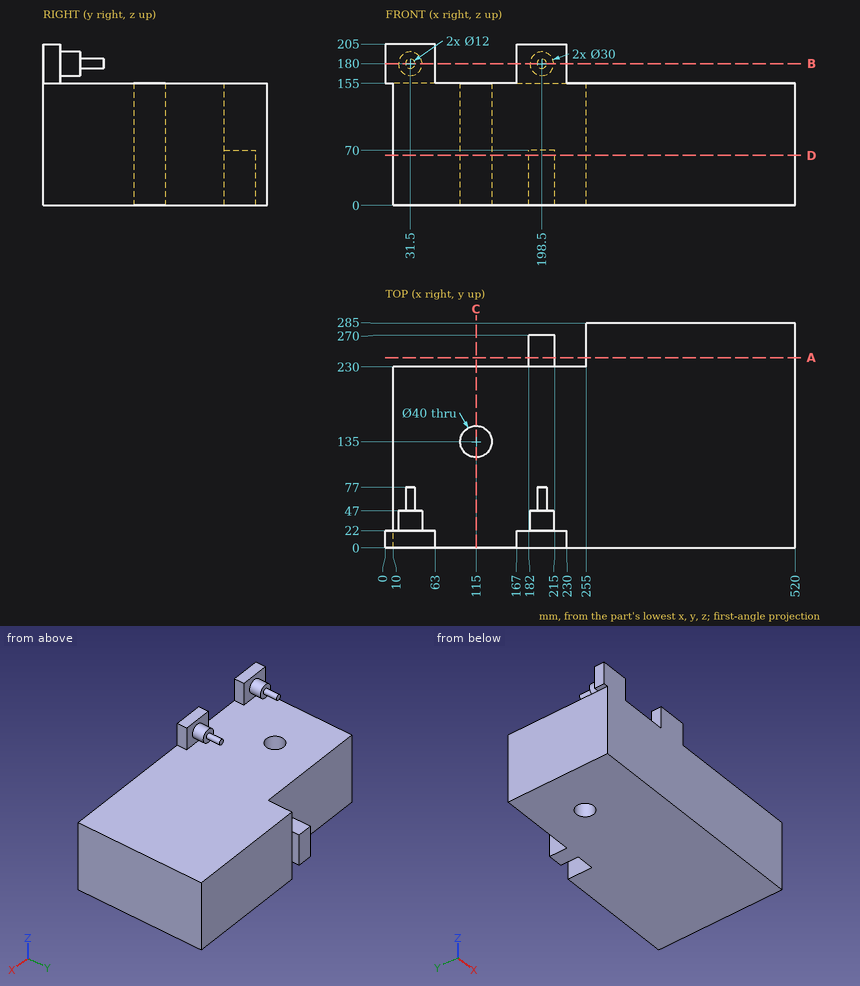
Here's the drawing with two shaded views (mm, measured from the low corner). I have some questions. Round coordinates to 2 decimals unless told otherwise and drop trailing zeros. Order: outer loops, then holes, each group sorted by start corner. A loop starts at its lowest first (then second) coordinate and runs counter-clockwise, first axis right, second up. Notation, with made-up numbers: (61, 85) -> (105, 85) arc R16 ccw to (105, 104) -> close; hole circle Ø8 at (73, 14). An arc over 180 degrees is marked (long way). Return JSON: item names as keys, results as strings.
Q1. If we section it at D-D on z = 63.5: List the corners of the cut face in (x, y) for me.
Filled sheet:
{"outline": "(10, 0) -> (520, 0) -> (520, 285) -> (255, 285) -> (255, 230) -> (215, 230) -> (215, 270) -> (182, 270) -> (182, 230) -> (10, 230) -> close; hole circle Ø40 at (115, 135)"}
Q2. I need wall thicknesses on line 1 along Y through (x, z) = (115, 75.5); line 2 along Z through (x, y) = (499.5, 121.5); line 3 along X through (y, z) = (201, 148.5). Which ranges of each line are inside material? Lowest first, please. Write a range as from..to.
Filled sheet:
{"line 1": "y = 0..115, 155..230", "line 2": "z = 0..155", "line 3": "x = 10..520"}
Q3. If we section it at A-A on y = 241.5: List the corners of the cut face in (x, z) for me, plus the area to 3 significant figures.
Filled sheet:
{"outline": "(182, 0) -> (215, 0) -> (215, 70) -> (182, 70) -> close; (255, 0) -> (520, 0) -> (520, 155) -> (255, 155) -> close", "area": "43,400 mm^2"}
Q4. For pin 1 Ø9.5 at (x, z) = (33, 178.5) entering from +Y; pin 2 Ø16.5 at (x, y) = (193.5, 255) entering from +Z; pin 3 Ø20 at (y, z) = (256.5, 23.5) entering from -X; pin 4 Ø3 at (x, z) = (237, 82) entering from -Y, each with a flat end and sliding along its axis, tell me the tip position at first contact or that it passes through.
Filled sheet:
{"pin 1": "stops at y = 77", "pin 2": "stops at z = 70", "pin 3": "stops at x = 182", "pin 4": "stops at y = 0"}
Q5. If we section it at C-C on x = 115: List the corners of the cut face in (y, z) for me, plus the area to 4 significant figures.
Filled sheet:
{"outline": "(0, 0) -> (115, 0) -> (115, 155) -> (0, 155) -> close; (155, 0) -> (230, 0) -> (230, 155) -> (155, 155) -> close", "area": "29,450 mm^2"}
Q6. If we section it at B-B on z = 180: List the corners of the cut face in (x, y) for me, plus the area to 3 significant figures.
Filled sheet:
{"outline": "(0, 0) -> (63, 0) -> (63, 22) -> (46.5, 22) -> (46.5, 47) -> (37.5, 47) -> (37.5, 77) -> (25.5, 77) -> (25.5, 47) -> (16.5, 47) -> (16.5, 22) -> (0, 22) -> close; (167, 0) -> (230, 0) -> (230, 22) -> (213.5, 22) -> (213.5, 47) -> (204.5, 47) -> (204.5, 77) -> (192.5, 77) -> (192.5, 47) -> (183.5, 47) -> (183.5, 22) -> (167, 22) -> close", "area": "4,990 mm^2"}
